For this review, take the finished solid that the model builds, in its own axes (mm). A direction names the side the tool comes from. Coordinates: 2 decimals unless noted, no trailing zeros. Order: outer loops, then holes, each group sorted by start corner. A loop starts at its lowest first (then second) coordinate and runs counter-clockwise, first axis right, second up. Notation, with made-up numbers: (28, 14) - (50, 14) arc R34 ccw to (50, 48) - close; hole circle Ø11 at (84.25, 50). An arc over 180 degrees is marked (long way). One line per item, written item: value. Start each with the question number.
(1) Consider section D-D on x = 50.5. Write out the cut boundary in (y, z), then the cut area to 3 significant figures.
(2) For faces 5 (the flat face through (-4.9, -1, -23)), 6 (the cylindrical face through (35.369, -1.479, 38.004)), 7 (the flat face through (-21, -1, 0)), list the 3-axis set-ups (+Z, -Z, +X, -X, +Y, -Y) from which the entire face can be reached by the end or side of a thin tool; tool diameter is ignored.
(3) Consider section C-C on z = 6.5. Write out the cut boundary in (x, y).
(4) Consider section A-A on x = -37. Write out the cut boundary in (y, z), then the cut area to 3 significant figures.
(5) Consider section B-B on y = -1.35. Write out the cut boundary in (x, z).
(6) Mouldability with a two-part tool opening along X and no side actions: class faces 1 (the flat face through (-34.096, -1, -23)), 2 (the flat face through (54.54, -1.48, 21.31)), 3 (the flat face through (1, -3, -8)), 4 (the cylindrical face through (-58.166, -1.479, -20.681)) as released by +X, released by -X, zero draft, split by the parting line, or undercut.
(7) To check wall thickness, follow line 1 along Z through (x, y) = (-2.5, -2.6); line 2 along Z through (x, y) = (-39.5, -2.4); line 3 along Z through (x, y) = (-31, -1.95). State the ranges of each line that lie inside material, in increasing order.
(8) Clearance check with flat-ended pins moving along their axes: pin 1 (0.9 mm diameter, centred on y = -1.5, z = -22.5, fed in from -X); pin 2 (3 mm diameter, centred on x = 19, z = -20.5, fed in from +Y); pin 3 (1.4 mm diameter, centred on y = -1.5, z = -22.5, fed in from +X); pin 4 (1.5 mm diameter, centred on y = -2, z = 15.5, fed in from +X). State where each tip first meets the part, or that it passes through.
```python
from build123d import *

# Parameters (mm, degrees)
F1_DEPTH = 3
F2_R     = 10
F3_W     = 4.9
F3_H     = 2.9
F4_DEPTH = 25
F5_DEPTH = 25


with BuildPart() as f1:
    # F0 (on Front) → F1 (new body)
    with BuildSketch(Plane.XZ):
        with BuildLine():
            ThreePointArc((-43.741338, 0), (-58.121657, -21.069105), (-38.998462, -37.951171))
            Line((-38.998462, -37.951171), (16.091859, -37.951171))
            Line((16.091859, -37.951171), (22.294076, -8.399412))
            Line((22.294076, -8.399412), (34.020763, 14.150426))
            Line((34.020763, 14.150426), (40.711638, 9.589177))
            Line((40.711638, 9.589177), (47.832642, 4.734704))
            ThreePointArc((47.832642, 4.734704), (58.386807, 0.478115), (61.229721, 11.497498))
            Line((61.229721, 11.497498), (47.663182, 31.398193))
            ThreePointArc((47.663182, 31.398193), (35.163182, 38.005054), (22.663182, 31.398193))
            Line((22.663182, 31.398193), (1.258662, 0))
            Line((1.258662, 0), (-43.741338, 0))
        make_face()
    extrude(amount=F1_DEPTH)

    # F2
    f2_edges = [f1.edges().sort_by_distance(p)[0] for p in [
        (16.091859, -1.5, -37.951171),
    ]]
    fillet(f2_edges, radius=F2_R)

    # F3 (on Front) → F4 (cut)
    with BuildSketch(Plane.XZ):
        with Locations((-36.54559, -22.766416)):
            Rectangle(F3_W, F3_H)
        with Locations((-2.45, -22.52518)):
            Rectangle(F3_W, F3_H)
    extrude(amount=-F4_DEPTH, mode=Mode.SUBTRACT)

    # F3 (on Front) → F5 (cut)
    with BuildSketch(Plane.XZ):
        with Locations((-36.54559, -22.766416)):
            Rectangle(F3_W, F3_H)
        with Locations((-2.45, -22.52518)):
            Rectangle(F3_W, F3_H)
    extrude(amount=F5_DEPTH, mode=Mode.SUBTRACT)


solid = f1.part
```
Geometry check:
1. outline: (-3, 1.13) - (0, 1.13) - (0, 27.24) - (-3, 27.24) - close
1. area: 78.3 mm^2
2. face 5: +Y, -Y
2. face 6: +Z, +Y, -Y
2. face 7: +Z, -X, +Y, -Y
3. outline: (5.69, -3) - (30.04, -3) - (30.04, 0) - (5.69, 0) - close; (45.24, -3) - (62.51, -3) - (62.51, 0) - (45.24, 0) - close
4. outline: (-3, -37.95) - (0, -37.95) - (0, -24.22) - (-3, -24.22) - close; (-3, -21.32) - (0, -21.32) - (0, 0) - (-3, 0) - close
4. area: 105 mm^2
5. outline: (-43.74, 0) arc R19.27 ccw to (-39, -37.95) - (7.97, -37.95) arc R10 ccw to (17.76, -30.01) - (22.29, -8.4) - (34.02, 14.15) - (47.83, 4.73) arc R7.57 ccw (long way) to (61.23, 11.5) - (47.66, 31.4) arc R15.13 ccw to (22.66, 31.4) - (1.26, 0) - close; hole (-39, -24.22) - (-34.1, -24.22) - (-34.1, -21.32) - (-39, -21.32) - close; hole (-4.9, -23.98) - (0, -23.98) - (0, -21.08) - (-4.9, -21.08) - close
6. face 1: undercut
6. face 2: released by +X
6. face 3: zero draft
6. face 4: released by -X
7. line 1: z = -37.95 to -23.98, -21.08 to 0
7. line 2: z = -37.94 to 0
7. line 3: z = -37.95 to 0
8. pin 1: stops at x = -57.97
8. pin 2: stops at y = 0
8. pin 3: stops at x = 19.48
8. pin 4: stops at x = 59.01
